Source: three-view drawing plus pictorial views. Frame: mm from the lowest corner of the part. A direction names the side the tool comes from. Round coordinates to 2 decimals unless told otherwise and drop trailing zeros. Order: outer loops, then holes, each group sorted by start corner. A loop starts at its lowest first (then second) coordinate and runs counter-clockwise, first axis right, second up. Notation, with made-up numbers: (28, 57.5) - (39, 57.5) arc R21 cw to (39, 66.5) - close; hole circle Ø5 at (80, 76.25). An arc over 180 degrees is marked (long way). Use one line per item in the form item = value. Start each with the question number.
Q1. Cut plane C-C, the plane x = 37. Return the cut outline in (y, z), and give its area (3 significant figures).
Q2. Cut plane B-B, the plane z = 50.5. Return the cut outline in (x, y).
Q3. Pin query (flat end, axial travel): pin 1 Ø3 at (x, y) = (93, 1.5) entering from -Z; pin 2 Ø19.5 at (x, z) = (89.5, 48.5) entering from +Y; pin 3 Ø6 at (y, z) = (3.5, 6.5) entering from +X; pin 4 Ø6 at (y, z) = (7.5, 15) entering from -X. Return the tip coordinate at first contact, or that it passes through.
Q4. Cut plane A-A, the plane y = 3.75. Return the cut outline in (x, z), and give its area (3 significant figures).
Q5. Cut plane D-D, the plane y = 17. Return the cut outline in (x, z).
Q6. Set-up query: the marked faces 1 and 2. Return all of +Z, -Z, +X, -X, +Y, -Y with unobstructed straight access to the full face (end or side cutting, diameter ignored); none if empty.
Q7. Ray query, line 1 (X direction, y = 12.5, z = 71.5); line 2 (Z direction, x = 20.5, y = 17); line 3 (X direction, y = 4.5, z = 5.5). Return the intervals inside material, ascending. Write a range as [from, to].
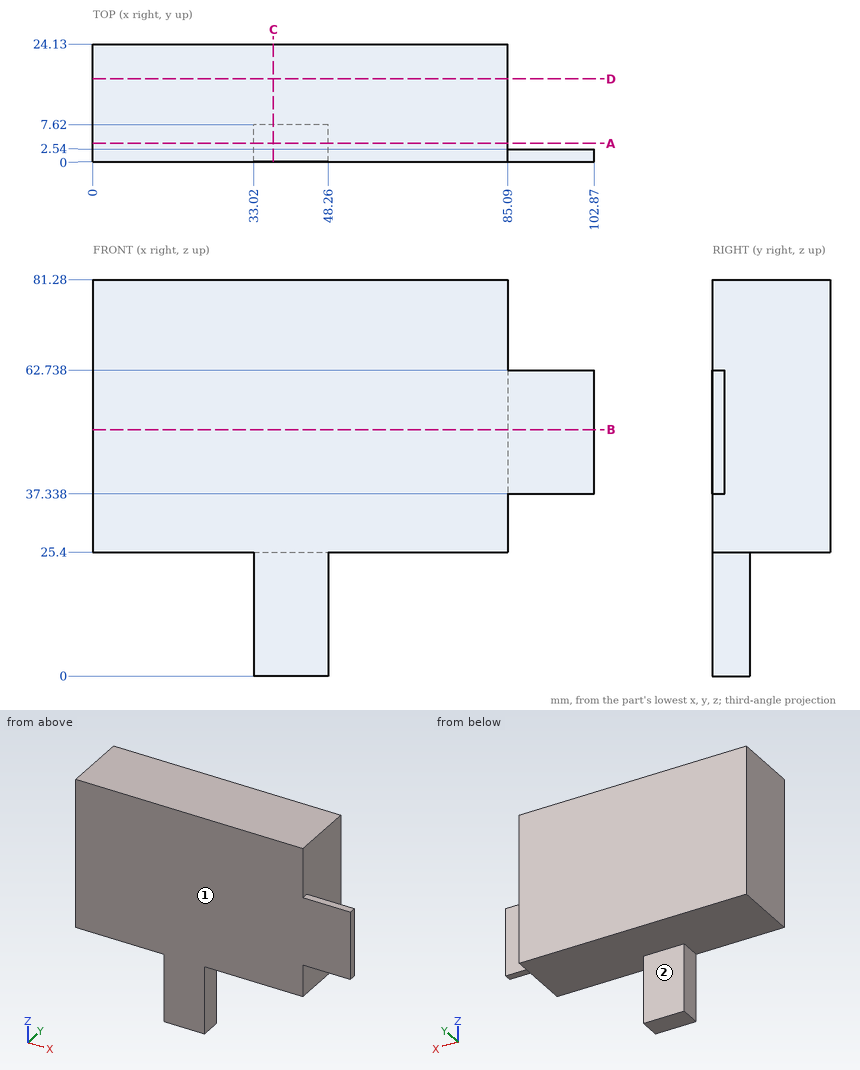
Completed:
q1.outline = (0, 0) - (7.62, 0) - (7.62, 25.4) - (24.13, 25.4) - (24.13, 81.28) - (0, 81.28) - close
q1.area = 1,540 mm2
q2.outline = (0, 0) - (102.87, 0) - (102.87, 2.54) - (85.09, 2.54) - (85.09, 24.13) - (0, 24.13) - close
q3.pin_1 = 37.34
q3.pin_2 = 24.13
q3.pin_3 = 48.26
q3.pin_4 = 33.02
q4.outline = (0, 25.4) - (33.02, 25.4) - (33.02, 0) - (48.26, 0) - (48.26, 25.4) - (85.09, 25.4) - (85.09, 81.28) - (0, 81.28) - close
q4.area = 5,140 mm2
q5.outline = (0, 25.4) - (85.09, 25.4) - (85.09, 81.28) - (0, 81.28) - close
q6.face_1 = +Z, -Z, +X, -X, -Y
q6.face_2 = -Z, +X, -X, +Y
q7.line_1 = [0, 85.09]
q7.line_2 = [25.4, 81.28]
q7.line_3 = [33.02, 48.26]
